For this review, use the dimensioned drawing (mm, ordinates from the lowest corner) and the shaded views. Give positions to 0.01 mm unless a question says otherwise; leave off trailing zeros. Order: outer loops, then holes, each group sorted by start corner. A loop starts at its lowest first (then second) coordinate and runs counter-clockwise, first axis right, second up.
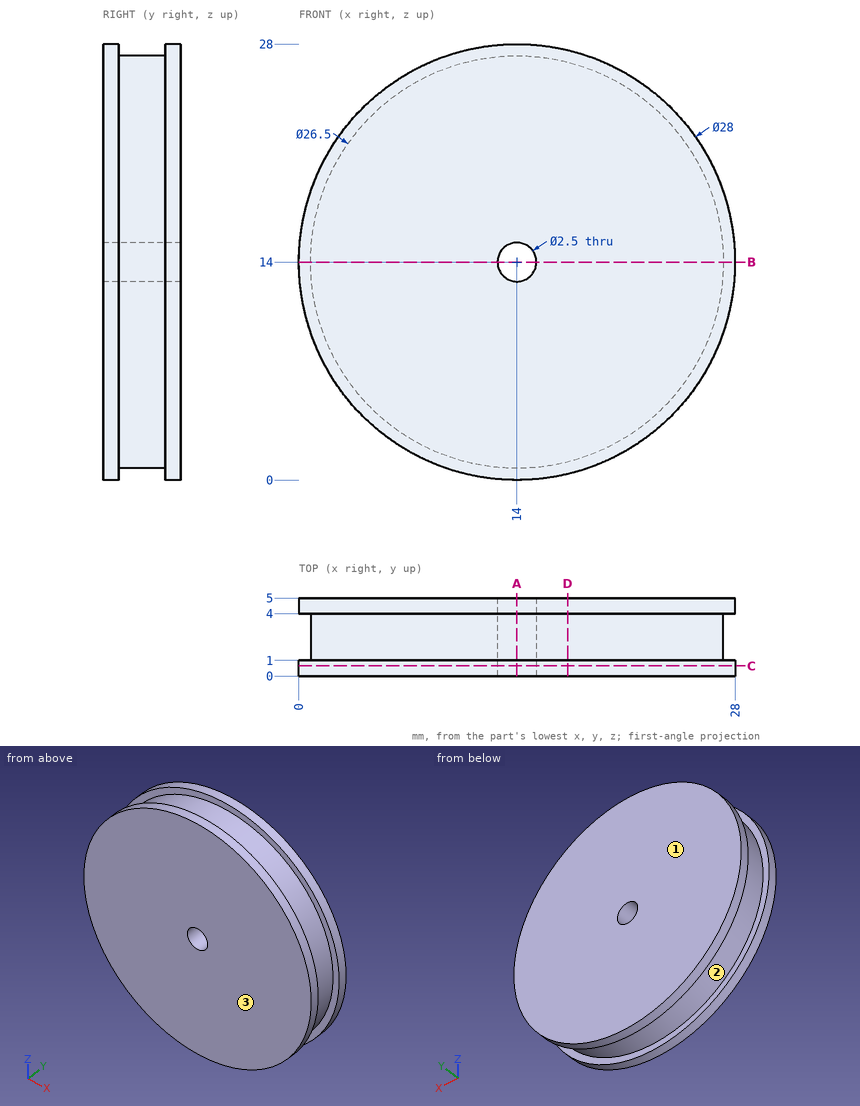
1. Take a section at A-A (x = 14). State the section outline as (y, z) points, then the cut area to 3 significant figures.
Recorded:
outline: (0, 0) - (1, 0) - (1, 0.75) - (4, 0.75) - (4, 0) - (5, 0) - (5, 12.75) - (0, 12.75) - close; (0, 15.25) - (5, 15.25) - (5, 28) - (4, 28) - (4, 27.25) - (1, 27.25) - (1, 28) - (0, 28) - close
area: 123 mm2
2. For line 1 along X through (y, z) = (1.4, 14); line 2 along Z through (x, y) = (14.5, 1.2), list the stretches that pass through material, from the lowest coordinate up.
Recorded:
line 1: x = 0.75 to 12.75, 15.25 to 27.25
line 2: z = 0.76 to 12.85, 15.15 to 27.24
3. Draft analysis for pull direction Y (two halves, no side actions). For the marked faces 1, 2 and 3, state which applies: pulls with the +Y half, pulls with the -Y half, needs draft (parallel to the pull), parting line crosses it, or undercut.
Recorded:
face 1: pulls with the +Y half
face 2: undercut
face 3: pulls with the -Y half
4. For pin 1 (2 mm diameter, centred on y = 2.5, z = 16, fed in from -X); pin 2 (2 mm diameter, centred on x = 18, y = 4, fed in from -Z); pin 3 (2 mm diameter, centred on x = 14, z = 14, fed in from -Y), all flat-tipped, find the tip position at first contact; note any pin that passes through.
Recorded:
pin 1: stops at x = 0.79
pin 2: stops at z = 0.33
pin 3: passes through
5. Take a section at B-B (z = 14). State the section outline as (x, y) points, then the cut area to 3 significant figures.
Recorded:
outline: (0, 0) - (12.75, 0) - (12.75, 5) - (0, 5) - (0, 4) - (0.75, 4) - (0.75, 1) - (0, 1) - close; (15.25, 0) - (28, 0) - (28, 1) - (27.25, 1) - (27.25, 4) - (28, 4) - (28, 5) - (15.25, 5) - close
area: 123 mm2
6. Take a section at C-C (y = 0.65). State the section outline as (x, z) points, then the cut area to 3 significant figures.
Recorded:
outline: circle Ø28 at (14, 14); hole circle Ø2.5 at (14, 14)
area: 611 mm2
7. Take a section at D-D (x = 17.25). State the section outline as (y, z) points, then the cut area to 3 significant figures.
Recorded:
outline: (0, 0.38) - (1, 0.38) - (1, 1.15) - (4, 1.15) - (4, 0.38) - (5, 0.38) - (5, 27.62) - (4, 27.62) - (4, 26.85) - (1, 26.85) - (1, 27.62) - (0, 27.62) - close
area: 132 mm2
